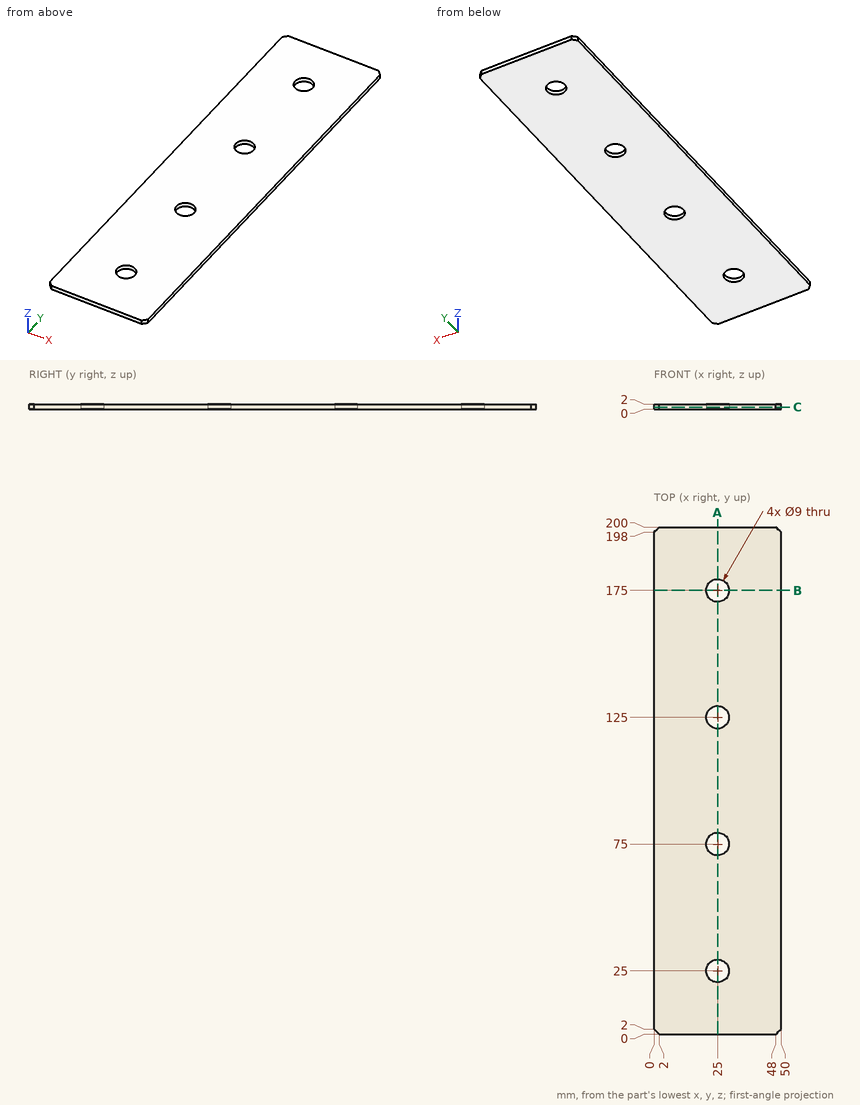
Answer from the drawing. Dimensions are ordinates in mm from the lowest x, y and z of the part. Coordinates: 2 decimals unless noted, no trailing zeros. Loops run counter-clockwise (first coordinate to the right, second up) from the corner with the lowest first, then second, coordinate; pieces in that order, holes last. Notation, with made-up numbers: (-39.75, -19) -> (14.25, -19) arc R28 cw to (14.25, 14) -> close; hole circle Ø2 at (-2.75, 84.25). An arc over 180 degrees is marked (long way). Return JSON: item names as keys, results as strings.
Item 1: Find section A-A (x = 25). Determine the outline of the cut face in (y, z).
Answers:
{"outline": "(0, 0) -> (20.5, 0) -> (20.5, 2) -> (0, 2) -> close; (29.5, 0) -> (70.5, 0) -> (70.5, 2) -> (29.5, 2) -> close; (79.5, 0) -> (120.5, 0) -> (120.5, 2) -> (79.5, 2) -> close; (129.5, 0) -> (170.5, 0) -> (170.5, 2) -> (129.5, 2) -> close; (179.5, 0) -> (200, 0) -> (200, 2) -> (179.5, 2) -> close"}
Item 2: Find section C-C (z = 0.8). Determine the outline of the cut face in (x, y), plus the area to 3 significant figures.
Answers:
{"outline": "(0, 2) -> (2, 0) -> (48, 0) -> (50, 2) -> (50, 198) -> (48, 200) -> (2, 200) -> (0, 198) -> close; hole circle Ø9 at (25, 25); hole circle Ø9 at (25, 75); hole circle Ø9 at (25, 125); hole circle Ø9 at (25, 175)", "area": "9,740 mm2"}
Item 3: A flat-ended cylindrical pin translates along its axis: P1, Ø14.5, axis at x = 25, y = 175, coming from the -Z side. Find the tip coordinate at first contact, or state that the pin passes through.
Answers:
{"P1": "stops at z = 0"}
Item 4: Find section B-B (y = 175). Determine the outline of the cut face in (x, z), plus the area to 3 significant figures.
Answers:
{"outline": "(0, 0) -> (20.5, 0) -> (20.5, 2) -> (0, 2) -> close; (29.5, 0) -> (50, 0) -> (50, 2) -> (29.5, 2) -> close", "area": "82.0 mm2"}
Item 5: Find the intervals of material crossed by probe 1 along Y at (x, z) = (25, 0.7); probe 2 along Y at (x, z) = (27.5, 1.4); probe 3 along X at (y, z) = (78.5, 1.6), in increasing order.
Answers:
{"probe 1": "y = 0 to 20.5, 29.5 to 70.5, 79.5 to 120.5, 129.5 to 170.5, 179.5 to 200", "probe 2": "y = 0 to 21.26, 28.74 to 71.26, 78.74 to 121.26, 128.74 to 171.26, 178.74 to 200", "probe 3": "x = 0 to 22.17, 27.83 to 50"}
